Part model, mm, in its own coordinate system. Give positions to 0.01 mm unless a question says otherwise; leave off trailing zeros. Order: outer loops, then holes, each group sorted by start corner. A loop starts at its lowest first (then second) coordinate and runs counter-clockwise, first axis right, second up. Notation, with made-up numbers: (-9, 4.25) - (31, 4.25) arc R20 cw to (31, 24.25) - close; hole circle Ø1 at (76.5, -14.5). An arc over 180 degrees is marked (long way). One line per item, written item: value.
```python
from build123d import *

# Parameters (mm, degrees)
RESSALTO_EXTRUS_O1_DEPTH = 0.2
RESSALTO_EXTRUS_O2_DEPTH = 0.2
CORTE_EXTRUS_O1_DEPTH    = 1
FILETE1_R                = 0.05
RESSALTO_EXTRUS_O3_DEPTH = 0.145
PADR_O_LINEAR1_COUNT     = 2
PADR_O_LINEAR1_PITCH     = 0.505
CORTE_EXTRUS_O2_DEPTH    = 0.3


with BuildPart() as part:
    # Esboço1 → Ressalto-extrusão1 (new body)
    with BuildSketch(Plane.XY):
        with BuildLine():
            Line((76.710328142, 206.616112347), (76.710328142, 206.416112347))
            Line((76.710328142, 206.416112347), (76.657349848, 206.416112347))
            Line((76.657349848, 206.416112347), (76.657349848, 206.116112347))
            Line((76.657349848, 206.116112347), (76.645328142, 206.116112347))
            Line((76.645328142, 206.116112347), (76.610328142, 206.116112347))
            Line((76.610328142, 206.116112347), (76.560328142, 206.116112347))
            ThreePointArc((76.560328142, 206.116112347), (76.524972803, 206.101467686), (76.510328142, 206.066112347))
            Line((76.510328142, 206.066112347), (76.510328142, 205.966112347))
            Line((76.510328142, 205.966112347), (76.110328142, 205.966112347))
            Line((76.110328142, 205.966112347), (76.081970009, 205.966112347))
            Line((76.081970009, 205.966112347), (75.910328142, 205.966112347))
            Line((75.910328142, 205.966112347), (75.595453106, 206.080717488))
            ThreePointArc((75.595453106, 206.080717488), (75.537376388, 206.073071543), (75.510328142, 206.021112347))
            Line((75.510328142, 206.021112347), (75.510328142, 205.971112347))
            Line((75.510328142, 205.971112347), (75.410328142, 205.971112347))
            Line((75.410328142, 205.971112347), (75.309933917, 206.02907498))
            ThreePointArc((75.309933917, 206.02907498), (75.273690046, 206.034493063), (75.243486264, 206.013739619))
            ThreePointArc((75.243486264, 206.013739619), (75.229104336, 206.000793024), (75.210328142, 205.996112347))
            Line((75.210328142, 205.996112347), (75.160328142, 205.996112347))
            Line((75.160328142, 205.996112347), (74.960328142, 206.041112347))
            Line((74.960328142, 206.041112347), (70.860328142, 206.041112347))
            Line((70.860328142, 206.041112347), (70.560328142, 206.141112347))
            Line((70.560328142, 206.141112347), (70.560328142, 206.391112347))
            Line((70.560328142, 206.391112347), (70.860328142, 206.491112347))
            Line((70.860328142, 206.491112347), (74.960328142, 206.491112347))
            Line((74.960328142, 206.491112347), (75.150344741, 206.536112347))
            Line((75.150344741, 206.536112347), (75.210328142, 206.536112347))
            ThreePointArc((75.210328142, 206.536112347), (75.229104336, 206.53143167), (75.243486264, 206.518485075))
            ThreePointArc((75.243486264, 206.518485075), (75.273690046, 206.497731631), (75.309933917, 206.503149714))
            Line((75.309933917, 206.503149714), (75.410328142, 206.561112347))
            Line((75.410328142, 206.561112347), (75.510328142, 206.561112347))
            Line((75.510328142, 206.561112347), (75.510328142, 206.511112347))
            ThreePointArc((75.510328142, 206.511112347), (75.540942979, 206.456830135), (75.60323487, 206.454946752))
            Line((75.60323487, 206.454946752), (75.910328142, 206.616112347))
            Line((75.910328142, 206.616112347), (76.081970009, 206.616112347))
            Line((76.081970009, 206.616112347), (76.110328142, 206.616112347))
            Line((76.110328142, 206.616112347), (76.710328142, 206.616112347))
        make_face()
    extrude(amount=RESSALTO_EXTRUS_O1_DEPTH)

    # Esboço2 → Ressalto-extrusão2 (add)
    with BuildSketch(Plane.XZ.offset(-206.416112347)):
        with BuildLine():
            Line((76.710328142, 0), (76.710328142, 0.2))
            ThreePointArc((76.710328142, 0.2), (76.851749499, 0.258578644), (76.910328142, 0.4))
            Line((76.910328142, 0.4), (76.910328142, 3.38))
            ThreePointArc((76.910328142, 3.38), (77.02748543, 3.662842712), (77.310328142, 3.78))
            Line((77.310328142, 3.78), (78.110328142, 3.78))
            Line((78.110328142, 3.78), (78.110328142, 3.58))
            Line((78.110328142, 3.58), (77.310328142, 3.58))
            ThreePointArc((77.310328142, 3.58), (77.168906786, 3.521421356), (77.110328142, 3.38))
            Line((77.110328142, 3.38), (77.110328142, 0.4))
            ThreePointArc((77.110328142, 0.4), (76.993170855, 0.117157288), (76.710328142, 0))
        make_face()
    extrude(amount=-RESSALTO_EXTRUS_O2_DEPTH)

    # Esboço3 → Corte-extrusão1 (cut)
    with BuildSketch(Plane(origin=(0, 206.491112347, 0), x_dir=(1, 0, 0), z_dir=(0, 1, 0))):
        Polygon((70.860328142, 0), (70.560328142, -0.1), (70.475949981, -0.1), (70.475949981, 0.09851766), (70.860328142, 0.09851766), align=None)
    extrude(amount=-CORTE_EXTRUS_O1_DEPTH, mode=Mode.SUBTRACT)

    # Filete1
    filete1_edges = [part.edges().sort_by_distance(p)[0] for p in [
        (78.110328142, 206.616112347, 3.68),
        (78.110328142, 206.416112347, 3.68),
    ]]
    fillet(filete1_edges, radius=FILETE1_R)

    # Esboço4 → Ressalto-extrusão3 (add)
    with BuildSketch(Plane(origin=(0, 206.616112347, 0), x_dir=(1, 0, 0), z_dir=(0, 1, 0))):
        Polygon((76.057628142, 0), (76.310328142, 0), (76.310328142, 0.0624), align=None)
    ressalto_extrus_o3 = extrude(amount=-RESSALTO_EXTRUS_O3_DEPTH)

    # Padrão linear1: Ressalto-extrusão3 ×2
    with Locations(*[(0, -i * PADR_O_LINEAR1_PITCH, 0) for i in range(1, PADR_O_LINEAR1_COUNT)]):
        add(ressalto_extrus_o3)

    # Esboço5 → Corte-extrusão2 (cut)
    with BuildSketch(Plane.XZ.offset(-206.116112347)):
        Polygon((76.657349848, 0.16), (76.645349848, 0.16), (76.608838995, 0.2), (76.608838995, 0.232444762), (76.679680574, 0.232444762), (76.679680574, 0.16), align=None)
        Polygon((76.608838995, 0), (76.645349848, 0.04), (76.679680574, 0.04), (76.679680574, -0.014078239), (76.608838995, -0.014078239), align=None)
    extrude(amount=-CORTE_EXTRUS_O2_DEPTH, mode=Mode.SUBTRACT)


solid = part.part
```
1) Wall check: line 1 along Y through (x, z) = (77, 1.65); line 2 along X through (y, z) = (206.45, 0.5); line 3 along Z through (x, y) = (71.75, 206.25). Give the ranges that are in metal, low to high. Write a range as [from, to].
Answer:
line 1: y = [206.42, 206.62]
line 2: x = [76.91, 77.11]
line 3: z = [0, 0.2]
2) Slice it at B-B on x = 77.5. Write the cut outline in (y, z).
Answer:
outline: (206.42, 3.58) - (206.62, 3.58) - (206.62, 3.78) - (206.42, 3.78) - close
3) Slice it at C-C on z = 2.35. Write the cut outline in (x, y), then the cut area to 3 significant figures.
Answer:
outline: (76.91, 206.42) - (77.11, 206.42) - (77.11, 206.62) - (76.91, 206.62) - close
area: 0.0400 mm2
